For this review, take the finished solid that the model builds, in its own axes (mm). Face numbers are marked on the shaded views. A direction names the side the tool comes from. Coordinates: 2 decimals unless noted, no trailing zeros. Loops run counter-clockwise (first coordinate to the right, second up) from the corner with the lowest first, then second, coordinate; pieces in that order, holes last. Notation, with made-up numbers: M 79.5,29.5 L 85.5,29.5 A33 ccw 85.5,65.5 Z; hole C 70,65 d1. An arc over 180 degrees is marked long. Put each result on its own line as item: value.
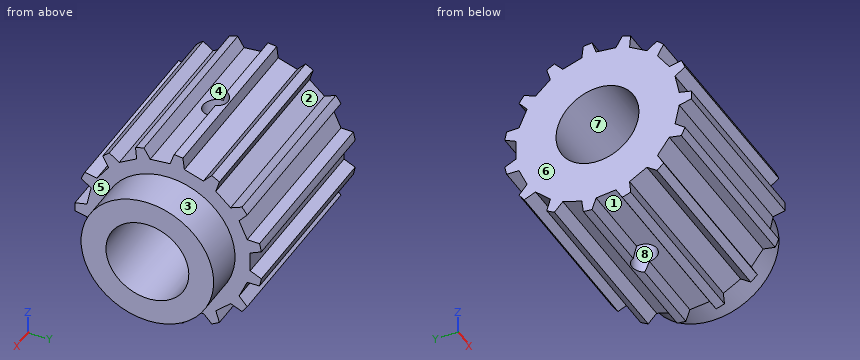
```python
from build123d import *

# Parameters (mm, degrees)
ENL_V_MAT_EXTRU_1_DEPTH      = 32.392853486
ENL_V_MAT_EXTRU_1_DEPTH_BACK = 32.392853486
ESQUISSE2_R                  = 1.5
ENL_V_MAT_EXTRU_2_REACH      = 33.393
R_P_TITION_CIRCULAIRE1_COUNT = 15


with BuildPart() as part:
    # Esquisse1 → Révolution1 (revolve)
    with BuildSketch(Plane.XY, mode=Mode.PRIVATE) as r_volution1_sk:
        Polygon((0, 5), (0, 8), (-5, 8), (-5, 11.325), (-27, 11.325), (-27, 5), align=None)
    revolve(r_volution1_sk.sketch.rotate(Axis((-12.25475793, 0, 0), (1, 0, 0)), 90), axis=Axis((-12.25475793, 0, 0), (1, 0, 0)))

    # Esquisse2 → Enlèv. mat.-Extru.1 (cut, two sides: drawn at the far end of the back side and taken through both)
    with BuildSketch(Plane.XY.offset(-ENL_V_MAT_EXTRU_1_DEPTH_BACK)):
        with Locations((-16, 0)):
            Circle(ESQUISSE2_R)
    extrude(amount=ENL_V_MAT_EXTRU_1_DEPTH + ENL_V_MAT_EXTRU_1_DEPTH_BACK, mode=Mode.SUBTRACT)

    # Esquisse3 → Enlèv. mat.-Extru.2 (cut, up to next)
    with BuildSketch(Plane.ZY.offset(27), mode=Mode.PRIVATE) as enl_v_mat_extru_2_sk1:
        with BuildLine():
            Line((-2.16, 11.88023674), (-1.204069301, 9.83023674))
            Line((-1.204069301, 9.83023674), (1.204069301, 9.83023674))
            Line((1.204069301, 9.83023674), (2.16, 11.88023674))
            ThreePointArc((2.16, 11.88023674), (0, 12.075), (-2.16, 11.88023674))
        make_face()
    enl_v_mat_extru_2_tool1 = extrude(enl_v_mat_extru_2_sk1.sketch, amount=-ENL_V_MAT_EXTRU_2_REACH, mode=Mode.PRIVATE) & part.part
    enl_v_mat_extru_2 = enl_v_mat_extru_2_tool1.solids().sort_by_distance((-27, 11.028097, 0))[0]
    add(enl_v_mat_extru_2, mode=Mode.SUBTRACT)

    # Répétition circulaire1: Enlèv. mat.-Extru.2 ×15 about axis
    r_p_tition_circulaire1_axis = Axis((0, 0, 0), (1, 0, 0))
    for i in range(1, R_P_TITION_CIRCULAIRE1_COUNT):
        add(enl_v_mat_extru_2.rotate(r_p_tition_circulaire1_axis, i * 360 / R_P_TITION_CIRCULAIRE1_COUNT), mode=Mode.SUBTRACT)


solid = part.part
```
(1) Draft analysis for pull direction X (two halves, no side actions). For the marked faces 5, 6, 7 and 8, state which applies: +X half, -X half, draft (parallel to the pull), parting line (faces both ways), or undercut.
Determined:
face 5: +X half
face 6: -X half
face 7: draft
face 8: undercut
(2) Add section D-D (y = 1). Write out the cut boundary in (x, z).
Determined:
outline: M -27,-11.28 L -17.12,-11.28 L -17.12,-4.9 L -27,-4.9 Z; M -27,4.9 L -17.12,4.9 L -17.12,11.28 L -27,11.28 Z; M -14.88,-11.28 L -5,-11.28 L -5,-7.94 L 0,-7.94 L 0,-4.9 L -14.88,-4.9 Z; M -14.88,4.9 L 0,4.9 L 0,7.94 L -5,7.94 L -5,11.28 L -14.88,11.28 Z
(3) Wall thickness on line 1 along X through (y, z) = (0, -7.75); line 2 along Y through (x, z) = (-7.5, 0) (3 decimals); line 3 along X through (y, z) = (0, 8.75): over which ranges is each line inside the solid? List them lowest first. Write a range as [from, to].
Determined:
line 1: x = [-27, -17.5], [-14.5, 0]
line 2: y = [-11.325, -5], [5, 9.83]
line 3: x = [-27, -17.5], [-14.5, -5]
(4) Add section A-A (z = 0). Write out the cut boundary in (x, y) (3 decimals), plus the area to 3 significant figures.
Determined:
outline: M -27,-11.325 L -5,-11.325 L -5,-8 L 0,-8 L 0,-5 L -27,-5 Z; M -27,5 L 0,5 L 0,8 L -5,8 L -5,9.83 L -27,9.83 Z
area: 275 mm^2
(5) Tool access review of the marked faces 1, 2, 3 and 4: name each direction out of +Z, -Z, +X, -X, +Y, -Y from which nothing blocks a thin tool from reaching the whole face with its end or side.
Determined:
face 1: -Z, +X, -X
face 2: +X, -X
face 3: +X
face 4: +Z, +X, -X
(6) Add section B-B (y = -3.5). Write out the cut boundary in (x, z), plus the area to 3 significant figures.
Determined:
outline: M -27,-10.77 L -5,-10.77 L -5,-7.19 L 0,-7.19 L 0,-3.57 L -27,-3.57 Z; M -27,3.57 L 0,3.57 L 0,7.19 L -5,7.19 L -5,10.77 L -27,10.77 Z
area: 353 mm^2
(7) Add section C-C (x = -1.75). Write out the cut boundary in (y, z), plus the area to 3 significant figures.
Determined:
outline: C 0,0 d16; hole C 0,0 d10
area: 123 mm^2
(8) For pin 1 (1 mm diameter, centred on x = -4, z = 4.5, fed in from +Y); pin 2 (8 mm diameter, centred on x = -21, z = 9, fed in from -Y); pin 3 (1 mm diameter, centred on x = -23.5, z = 4, fed in from +Y); pin 4 (2.5 mm diameter, centred on x = -16, y = 0, fed in from -Z), all flat-tipped, find the tip position at first contact; note any pin that passes through.
Determined:
pin 1: stops at y = 6.93
pin 2: stops at y = -10.16
pin 3: stops at y = 9.2
pin 4: passes through
